For this review, use the dimensioned drawing (mm, ordinates from the lowest corner) and the shaded views. A direction names the side the tool comes from. Give positions to 0.01 mm unless a question says otherwise; leave off trailing zeros. Loops run counter-clockwise (first coordinate to the right, second up) from the corner with the lowest first, then second, coordinate; pieces in that order, holes last. Notation, with made-up numbers: M -12.5,-18.5 L 21.5,-18.5 A21 ccw 21.5,-10.5 Z; hole C -8,-20.75 d11. An arc over 180 degrees is marked long. Use a Markdown table: item, result. Add a question column.
(1) For the marked faces 5 and 6, list the 3-axis set-ups (+Z, -Z, +X, -X, +Y, -Y) from which the entire face can be reached by the end or side of a thin tool; tool diameter is ignored.
(2) Draft analysis for pull direction X (two halves, no side actions). For the marked faces 1, 2, 3 and 4, state which applies: pulls with the +X half, pulls with the -X half, needs draft (parallel to the pull), parting line crosses it, or undercut.
(3) For probe 1 along X at (y, z) = (24.5, 41) (1 decimal); probe 2 along Y at (x, z) = (67, 82) (1 decimal); probe 3 along X at (y, z) = (38.5, 96), list the stretches that pass through material, from the lowest coordinate up.
(4) Insertion check: pin 1 Ø2 at (y, z) = (39, 104.5) entering from +X; pin 2 Ø1 at (x, y) = (34.5, 39.5) entering from -Z; pin 3 Ø12 at (x, z) = (43.5, 91) entering from -Y. Each pin has a flat end and moves straight along its axis. Give the tip position at first contact, or say it passes through.
(5) Add section D-D, the plane x = 37. Give the boundary of the cut face in (y, z) (1 decimal), then the cut area to 3 significant figures.
(6) Add section A-A, the plane y = 25. Give the boundary of the cut face in (x, z) (1 decimal).
(7) Add section B-B, the plane z = 15.5. Give the boundary of the cut face in (x, y) (1 decimal).
(8) Add section C-C, the plane z = 86. Give the boundary of the cut face in (x, y) (1 decimal).
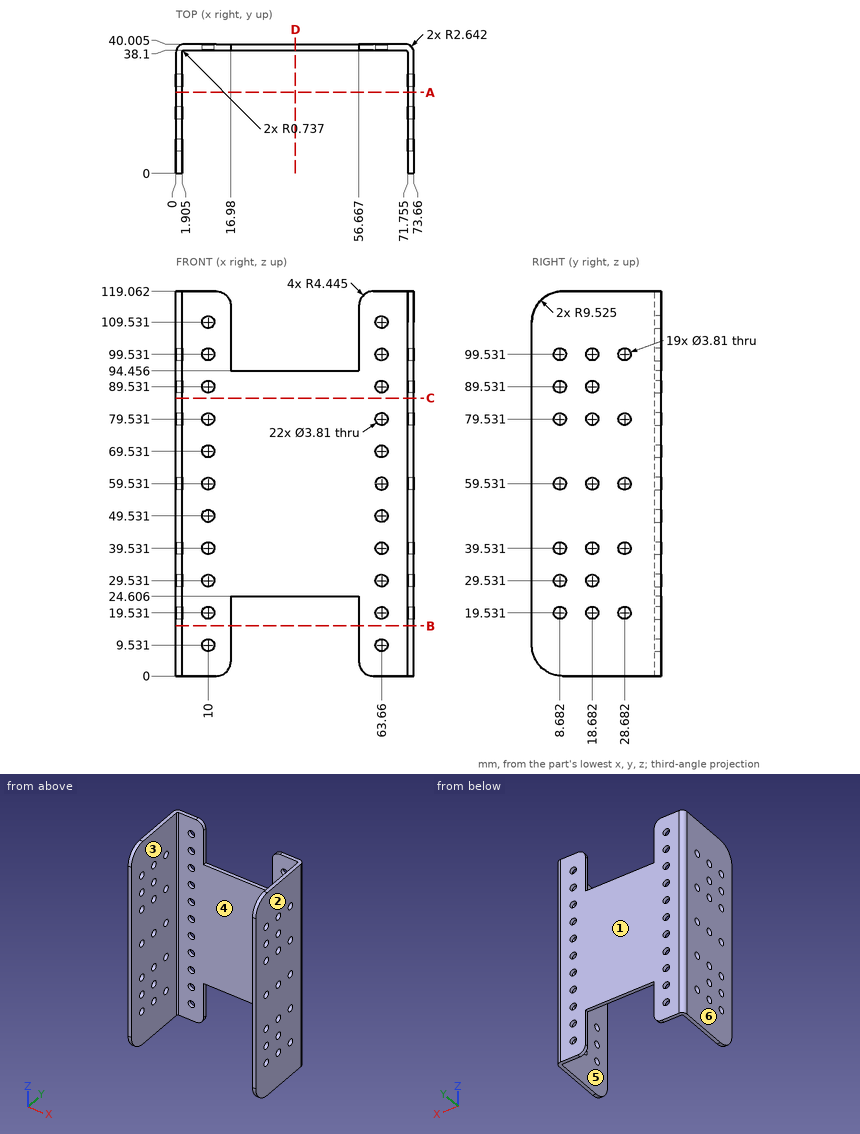
Established:
| question | item | result |
|---|---|---|
| 1 | face 5 | +Z, -Z, -Y |
| 1 | face 6 | +Z, -Z, -X, +Y, -Y |
| 2 | face 1 | needs draft |
| 2 | face 2 | pulls with the +X half |
| 2 | face 3 | undercut |
| 2 | face 4 | undercut |
| 3 | probe 1 | 0 to 1.9, 71.8 to 73.7 |
| 3 | probe 2 | 38.1 to 40 |
| 3 | probe 3 | 0.26 to 16.98, 56.67 to 73.4 |
| 4 | pin 1 | x = 73.58 |
| 4 | pin 2 | z = 24.61 |
| 4 | pin 3 | y = 38.1 |
| 5 | outline | M 38.1,24.6 L 40,24.6 L 40,94.5 L 38.1,94.5 Z |
| 5 | area | 133 mm^2 |
| 6 | outline | M 0,0 L 1.9,0 L 1.9,119.1 L 0,119.1 Z; M 71.8,0 L 73.7,0 L 73.7,119.1 L 71.8,119.1 Z |
| 7 | outline | M 0,0 L 1.9,0 L 1.9,37.4 A0.7 cw 2.6,38.1 L 17,38.1 L 17,40 L 2.6,40 A2.6 ccw 0,37.4 Z; M 56.7,38.1 L 71,38.1 A0.7 cw 71.8,37.4 L 71.8,0 L 73.7,0 L 73.7,37.4 A2.6 ccw 71,40 L 56.7,40 Z |
| 8 | outline | M 0,0 L 1.9,0 L 1.9,37.4 A0.7 cw 2.6,38.1 L 71,38.1 A0.7 cw 71.8,37.4 L 71.8,0 L 73.7,0 L 73.7,37.4 A2.6 ccw 71,40 L 2.6,40 A2.6 ccw 0,37.4 Z |
